Design review of the part built by this model. Coordinates are the model's own, in mm. Face numbers are marked on the shaded views. A direction names the side the tool comes from. Coordinates: 2 decimals unless noted, no trailing zeros. Loops run counter-clockwise (first coordinate to the right, second up) from the corner with the lowest first, then second, coordinate; pieces in that order, holes last. Notation, with made-up numbers: M -9,-39 L 25,-39 A23 cw 25,-1 Z; hole C -34,45.5 d6. An arc over 180 degrees is marked long. Put each result on its own line as item: value. Start each with the question number.
(1) Take a section at B-B, the plane x = -25.4. Give the boundary of the cut face in (y, z).
(2) Take a section at C-C, the plane z = 43.5. Give the boundary of the cut face in (x, y).
(3) Take a section at D-D, the plane x = -64. Give the boundary of the cut face in (y, z), then the cut area to 3 significant figures.
(4) Take a section at A-A, the plane y = 0. Give the boundary of the cut face in (x, z), then the cut area to 3 significant figures.
(5) For the marked faces 4 and 5, list the 3-axis set-ups (+Z, -Z, +X, -X, +Y, -Y) from which the entire face can be reached by the end or side of a thin tool; tool diameter is ignored.
(6) For probe 1 along Y at (x, z) = (-25.4, 42); probe 2 along X at (y, z) = (0, -24); probe 3 along Y at (x, z) = (-25.4, 110.5), list the stretches that pass through material, from the lowest coordinate up. Write a range as [from, to].
(7) Clearance check with flat-ended pins moving along their axes: pin 1 (6 mm diameter, centred on x = -51.5, z = -55.5, fed in from +Y); pin 2 (10 mm diameter, centred on y = 20, z = -55.5, fed in from +X); pin 3 (2 mm diameter, centred on x = -42, z = -81, fed in from +Y). State where each tip first meets the part, or that it passes through.
(8) The part is to be moulded in two halves that separate along X. For the marked faces 1, 2 and 3, say which applies: +X half, -X half, draft (parallel to the pull), parting line (faces both ways), or undercut.
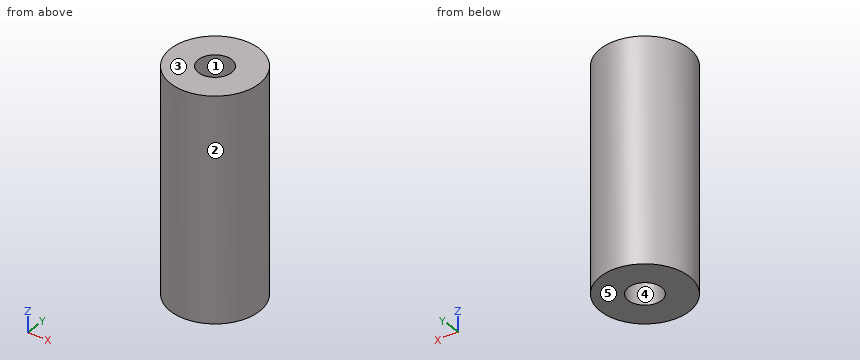
```python
from build123d import *

# Parameters (mm, degrees)
F0_W     = 38.1
F0_H     = 254
F2_R     = 19.05
F2_R_2   = 12.7
F3_DEPTH = 38.1
F4_R     = 19.05
F5_DEPTH = 38.1


with BuildPart() as f1:
    # F0 (on Front) → F1 (revolve)
    with BuildSketch(Plane.XZ):
        with Locations((6.35, 0)):
            Rectangle(F0_W, F0_H)
    revolve(axis=Axis((-25.4, 0, 0), (0, 0, -1)))

    # F2 (on face) → F3 (cut)
    with BuildSketch(Plane(origin=(0, 0, -127), x_dir=(1, 0, 0), z_dir=(0, 0, -1))):
        with Locations((-25.4, 0)):
            Circle(F2_R)
        with Locations((-25.4, 0)):
            Circle(F2_R_2, mode=Mode.SUBTRACT)
    extrude(amount=-F3_DEPTH, mode=Mode.SUBTRACT)

    # F4 (on face) → F5 (cut)
    with BuildSketch(Plane.XY.offset(127)):
        with Locations((-25.4, 0)):
            Circle(F4_R)
    extrude(amount=-F5_DEPTH, mode=Mode.SUBTRACT)


solid = f1.part
```
Computed values:
1. outline: M -50.8,-127 L -19.05,-127 L -19.05,-88.9 L -12.7,-88.9 L -12.7,88.9 L -19.05,88.9 L -19.05,127 L -50.8,127 Z; M 12.7,-88.9 L 19.05,-88.9 L 19.05,-127 L 50.8,-127 L 50.8,127 L 19.05,127 L 19.05,88.9 L 12.7,88.9 Z
2. outline: C -25.4,0 d101.6; hole C -25.4,0 d25.4
3. outline: M -33.03,-127 L 33.03,-127 L 33.03,127 L -33.03,127 Z
3. area: 16,800 mm^2
4. outline: M -76.2,-127 L -44.45,-127 L -44.45,-88.9 L -38.1,-88.9 L -38.1,88.9 L -44.45,88.9 L -44.45,127 L -76.2,127 Z; M -12.7,-88.9 L -6.35,-88.9 L -6.35,-127 L 25.4,-127 L 25.4,127 L -6.35,127 L -6.35,88.9 L -12.7,88.9 Z
4. area: 18,400 mm^2
5. face 4: -Z
5. face 5: -Z, +X, -X, +Y, -Y
6. probe 1: y = [-50.8, -12.7], [12.7, 50.8]
6. probe 2: x = [-76.2, -38.1], [-12.7, 25.4]
6. probe 3: y = [-50.8, -19.05], [19.05, 50.8]
7. pin 1: stops at y = 45.24
7. pin 2: stops at x = 23.13
7. pin 3: stops at y = 48.35
8. face 1: undercut
8. face 2: parting line
8. face 3: draft
